Geometry check sheet. Reference: the model listing, model coordinates, mm. Face numbers are marked on the shaded views. A direction names the side the tool comes from. Round coordinates to 2 decimals unless told otherwise and drop trailing zeros. Write each loop counter-clockwise with the first axis right and the second up, starting at its lowest first coordinate (ties: lowest second). Pieces come first, ordered by that corner, then holes. Notation, with made-up numbers: (22.25, 67.5) - (78.25, 67.5) arc R13 cw to (78.25, 79.5) - close; hole circle Ø5 at (-13, -2.5). An arc over 180 degrees is marked (long way). One line per question, with ' | ' between items. Start each with the question number.
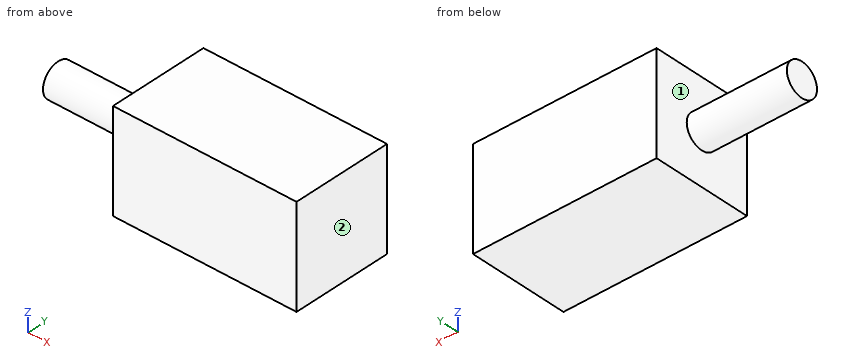
from build123d import *

# Parameters (mm, degrees)
BOSS_EXTRUDE1_DEPTH      = 19.05
BOSS_EXTRUDE1_DEPTH_BACK = 19.05
SKETCH1_W                = 69.85
SKETCH1_H                = 38.1
SKETCH3_W                = 38.1
SKETCH3_H                = 6.35


with BuildPart() as part:
    # Sketch1 → Boss-Extrude1 (new, two sides: drawn at the far end of the back side and taken through both)
    with BuildSketch(Plane(origin=(0, 0, 0), x_dir=(1, 0, 0), z_dir=(0, 1, 0)).offset(-BOSS_EXTRUDE1_DEPTH_BACK)):
        with Locations((34.925, 0)):
            Rectangle(SKETCH1_W, SKETCH1_H)
    extrude(amount=BOSS_EXTRUDE1_DEPTH + BOSS_EXTRUDE1_DEPTH_BACK)

    # Sketch3 → Revolve1 (revolve)
    with BuildSketch(Plane(origin=(0, 0, 0), x_dir=(1, 0, 0), z_dir=(0, 1, 0))):
        with Locations((-19.05, 3.175)):
            Rectangle(SKETCH3_W, SKETCH3_H)
    revolve(axis=Axis((0, 0, 0), (-1, 0, 0)))


solid = part.part
Q1. Set-up check for the marked faces 1 and 2: record each of +Z, -Z, +X, -X, +Y, -Y from which the full face is reachable in a straight line by a thin tool's end or side.
Q2. Section check A-A, the plane y = 0. Record the cut outline in (x, z).
Q3. Section check C-C, the plane y = 10. Record the cut outline in (x, z), then the cut area to 3 significant figures.
Q4. Go/stop test with flat-tipped pins: P1, Ø2, axis at x = -24.5, y = 3, coming from the -Z side; P2, Ø3, axis at y = 9.5, z = 0, coming from the -X side; P3, Ø8, axis at x = -12.5, z = -7.5, coming from the +Y side. Record where each tip stops, or that it passes through.
Q5. Thickness scan on line 1 (X direction, y = 16, z = 17); line 2 (Z direction, x = -8, y = 2.5). Record the ranges inside material, lowest first.
Result sheet:
1) face 1: -X | face 2: +Z, -Z, +X, +Y, -Y
2) outline: (-38.1, -6.35) - (0, -6.35) - (0, -19.05) - (69.85, -19.05) - (69.85, 19.05) - (0, 19.05) - (0, 6.35) - (-38.1, 6.35) - close
3) outline: (0, -19.05) - (69.85, -19.05) - (69.85, 19.05) - (0, 19.05) - close | area: 2,660 mm²
4) P1: z = -6.03 | P2: x = 0 | P3: y = 5.3
5) line 1: 0 to 69.85 | line 2: -5.84 to 5.84
